Verification items for the finished model (mm, model axes). Face numbers are marked on the shaded views. A direction names the side the tool comes from. Round coordinates to 2 decimals unless told otherwise and drop trailing zeros. Loops run counter-clockwise (first coordinate to the right, second up) from the corner with the lowest first, then second, coordinate; pieces in that order, holes last. Notation, with made-up numbers: (54.25, 61) -> (74.25, 61) arc R16 cw to (74.25, 87) -> close; hole circle Ø4 at (58, -28). An arc over 180 degrees is marked (long way). Write item = value, one per line. Start each with the question number.
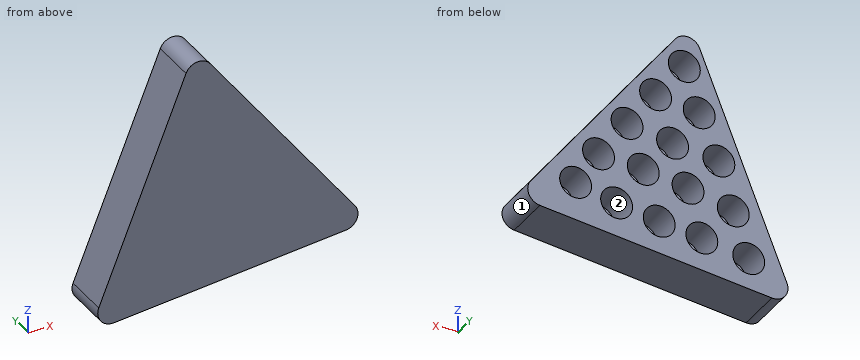
```python
from build123d import *

# Parameters (mm, degrees)
F1_DEPTH = 17.78
F2_R     = 5.08
F4_R     = 5.715
F5_DEPTH = 12.7


with BuildPart() as f1:
    # F0 (on Front) → F1 (new body)
    with BuildSketch(Plane.XZ):
        Polygon((-4.068127, 56.574355), (-41.914549, -37.713546), (58.66438, -23.345558), align=None)
    extrude(amount=F1_DEPTH)

    # F2
    f2_edges = [f1.edges().sort_by_distance(p)[0] for p in [
        (-4.068127, -8.89, 56.574355),
        (58.66438, -8.89, -23.345558),
        (-41.914549, -8.89, -37.713546),
    ]]
    fillet(f2_edges, radius=F2_R)

    # F4 (on face) → F5 (cut)
    with BuildSketch(Plane(origin=(0, 0, 0), x_dir=(-1, 0, 0), z_dir=(0, 1, 0))):
        with Locations((1.840184, 40.36641)):
            Circle(F4_R)
        with Locations((-8.471368, 27.190541)):
            Circle(F4_R)
        with Locations((7.1608, 24.728628)):
            Circle(F4_R)
        with Locations((-18.710878, 13.917103)):
            Circle(F4_R)
        with Locations((-2.386934, 10.979893)):
            Circle(F4_R)
        with Locations((14.226123, 8.879391)):
            Circle(F4_R)
        with Locations((-12.889439, -1.43216)):
            Circle(F4_R)
        with Locations((3.150751, -4.105525)):
            Circle(F4_R)
        with Locations((19.381898, -8.115573)):
            Circle(F4_R)
        with Locations((-22.437172, -16.326623)):
            Circle(F4_R)
        with Locations((-7.1608, -18.999988)):
            Circle(F4_R)
        with Locations((8.115572, -21.100491)):
            Circle(F4_R)
        with Locations((-28.92963, 0)):
            Circle(F4_R)
        with Locations((-37.140679, -12.698484)):
            Circle(F4_R)
        with Locations((24.919583, -24.155764)):
            Circle(F4_R)
    extrude(amount=-F5_DEPTH, mode=Mode.SUBTRACT)


solid = f1.part
```
(1) Section check B-B on x = 10.5. Enter the section's corners in (y, z), then the cut area to 3 significant figures.
(2) Section check A-A on y = -14. Enter the section's corners in (x, z).
(3) Section check C-C on z = 38. Enter the section's corners in (x, y), then the cut area to 3 significant figures.
(4) Depth check by flat-ended pin: pin 1 Ø8 at (y, z) = (-11.5, 26) entering from +X; pin 2 Ø5.5 at (x, z) = (39.5, -11.5) entering from +Y; pin 3 Ø8 at (y, z) = (-14, 34.5) entering from -X. Enter the tip coordinate at first touch or a pass-through.
(5) Access from +Z, -Z, +X, -X, +Y, -Y to the whole of each face (thin tool, end or side, straight path). Record for the marked faces 1 and 2.
(6) Scan lines: line 1 (Z direction, x = 9, y = -5); line 2 (X direction, y = -4.5, z = -4.5); line 3 (X direction, y = -0.75, z = -10.5). Record each from-to range of solid material in increasing order. Write a range as [from, to].
(7) Section check D-D on z = 0. Enter the section's corners in (x, y), then the cut area to 3 significant figures.
Computed values:
q1.outline = (-17.78, -30.23) -> (0, -30.23) -> (0, -23.64) -> (-12.7, -23.64) -> (-12.7, -14.36) -> (0, -14.36) -> (0, -6.62) -> (-12.7, -6.62) -> (-12.7, 3.76) -> (0, 3.76) -> (0, 21.85) -> (-12.7, 21.85) -> (-12.7, 32.53) -> (0, 32.53) -> (0, 38.01) -> (-17.78, 38.01) -> close
q1.area = 828 mm²
q2.outline = (-38.64, -29.55) arc R5.08 ccw to (-33.2, -36.47) -> (49.95, -24.59) arc R5.08 ccw to (53.23, -16.42) -> (1.36, 49.65) arc R5.08 ccw to (-7.35, 48.41) -> close
q3.outline = (-11.52, -17.78) -> (10.51, -17.78) -> (10.51, 0) -> (3.36, 0) -> (3.36, -12.7) -> (-7.04, -12.7) -> (-7.04, 0) -> (-11.52, 0) -> close
q3.area = 260 mm²
q4.pin_1 = 23.07
q4.pin_2 = -12.7
q4.pin_3 = -14.53
q5.face_1 = +X, +Y, -Y
q5.face_2 = +Y
q6.line_1 = [-30.44, -24.41], [-13.59, -5.62], [2.76, 21.5], [32.88, 39.93]
q6.line_2 = [-28.58, -23.81], [-14.96, -8.85], [2.55, 8.07], [17.71, 25.41], [32.45, 43.87]
q6.line_3 = [-30.99, -24.58], [-14.19, 31.87], [42.42, 48.58]
q7.outline = (-26.78, -17.78) -> (40.34, -17.78) -> (40.34, 0) -> (34.64, 0) -> (34.64, -12.7) -> (23.21, -12.7) -> (23.21, 0) -> (18.42, 0) -> (18.42, -12.7) -> (7.36, -12.7) -> (7.36, 0) -> (0.82, 0) -> (0.82, -12.7) -> (-7.13, -12.7) -> (-7.13, 0) -> (-26.78, 0) -> close
q7.area = 807 mm²
